Check sheet for the modelled part. Datum: model origin and axes. Units: mm. Give positions to 0.01 mm unless a question says otherwise; leave off trailing zeros. Order: outer loops, then holes, each group sorted by start corner. A loop starts at its lowest first (then second) coordinate and runs counter-clockwise, first axis right, second up.
Item 1: Sectioned sample at C-C on z = 0.05. Record the boundary of the cut face in (x, y) (1 decimal), and give its area (3 significant figures).
Item 2: Sectioned sample at D-D on x = 42. Record the boundary of the cut face in (y, z), and give its area (3 significant figures).
Item 3: Material ranges on line 1 along Y through (x, z) = (26, 0.05) (1 decimal), recorded low to high.
Item 4: Sectioned sample at B-B on x = 46.5. Record the boundary of the cut face in (y, z).
Item 5: Sectioned sample at A-A on y = -26.5. Record the boundary of the cut face in (x, z), and give its area (3 significant figures).
from build123d import *

# Parameters (mm, degrees)
MODEL_W                 = 8.2
MODEL_H                 = 3
SALIENTE_EXTRUIR1_DEPTH = 0.1


with BuildPart() as part:
    # Model → Saliente-Extruir1 (new body)
    with BuildSketch(Plane.XY):
        with BuildLine():
            Line((38.133331438, 3.018818363), (57.179927809, 5.173191598))
            ThreePointArc((57.179927809, 5.173191598), (56.564184394, 2.876430864), (55.882023409, 0.598513786))
            ThreePointArc((55.882023409, 0.598513786), (56.320793695, -11.111458732), (54.141567414, -22.625230857))
            ThreePointArc((54.141567414, -22.625230857), (54.328024919, -24.933799392), (53.741439305, -27.174373514))
            ThreePointArc((53.741439305, -27.174373514), (47.17770756, -29.193874015), (40.314312824, -28.959845377))
            ThreePointArc((40.314312824, -28.959845377), (40.492148067, -25.099981333), (40.891508653, -21.256716194))
            ThreePointArc((40.891508653, -21.256716194), (40.199471936, -10.428965006), (39.796709943, 0.413400668))
            ThreePointArc((39.796709943, 0.413400668), (38.077330395, 1.62185217), (36.383150384, 0.378318835))
            ThreePointArc((36.383150384, 0.378318835), (35.993185815, -10.447336237), (35.292291091, -21.257314345))
            ThreePointArc((35.292291091, -21.257314345), (35.69426102, -25.128822948), (35.871435139, -29.017108947))
            ThreePointArc((35.871435139, -29.017108947), (29.002751827, -29.224427494), (22.443184445, -27.176534138))
            ThreePointArc((22.443184445, -27.176534138), (21.856306031, -24.936090235), (22.042444158, -22.627547891))
            ThreePointArc((22.042444158, -22.627547891), (19.872780358, -11.081256605), (20.328112859, 0.658290054))
            ThreePointArc((20.328112859, 0.658290054), (19.658091011, 2.85533825), (19.057482139, 5.072367576))
            Line((19.057482139, 5.072367576), (38.133331438, 3.018818363))
        make_face()
        with Locations((28.59004178, -20.657297672)):
            Rectangle(MODEL_W, MODEL_H, mode=Mode.SUBTRACT)
        with Locations((47.59004178, -20.657297672)):
            Rectangle(MODEL_W, MODEL_H, mode=Mode.SUBTRACT)
    extrude(amount=SALIENTE_EXTRUIR1_DEPTH)


solid = part.part
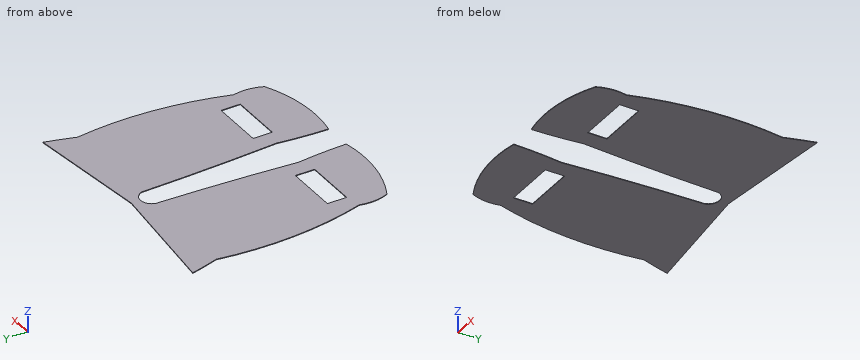
Report:
1. outline: (19.1, 5.1) arc R73 ccw to (20.3, 0.7) arc R52.4 ccw to (22, -22.6) arc R6.9 ccw to (22.4, -27.2) arc R20.7 ccw to (35.9, -29) arc R67.2 ccw to (35.3, -21.3) arc R376.9 ccw to (36.4, 0.4) arc R1.8 cw to (39.8, 0.4) arc R406.4 ccw to (40.9, -21.3) arc R67.2 ccw to (40.3, -29) arc R20.7 ccw to (53.7, -27.2) arc R6.9 ccw to (54.1, -22.6) arc R52.3 ccw to (55.9, 0.6) arc R81.9 ccw to (57.2, 5.2) - (38.1, 3) - close; hole (24.5, -22.2) - (32.7, -22.2) - (32.7, -19.2) - (24.5, -19.2) - close; hole (43.5, -22.2) - (51.7, -22.2) - (51.7, -19.2) - (43.5, -19.2) - close
1. area: 970 mm2
2. outline: (-29.23, 0) - (3.46, 0) - (3.46, 0.1) - (-29.23, 0.1) - close
2. area: 3.27 mm2
3. line 1: y = -28.6 to -22.2, -19.2 to 4.3
4. outline: (-29.27, 0) - (-22.16, 0) - (-22.16, 0.1) - (-29.27, 0.1) - close; (-19.16, 0) - (3.97, 0) - (3.97, 0.1) - (-19.16, 0.1) - close
5. outline: (22.18, 0) - (35.78, 0) - (35.78, 0.1) - (22.18, 0.1) - close; (40.4, 0) - (54, 0) - (54, 0.1) - (40.4, 0.1) - close
5. area: 2.72 mm2
